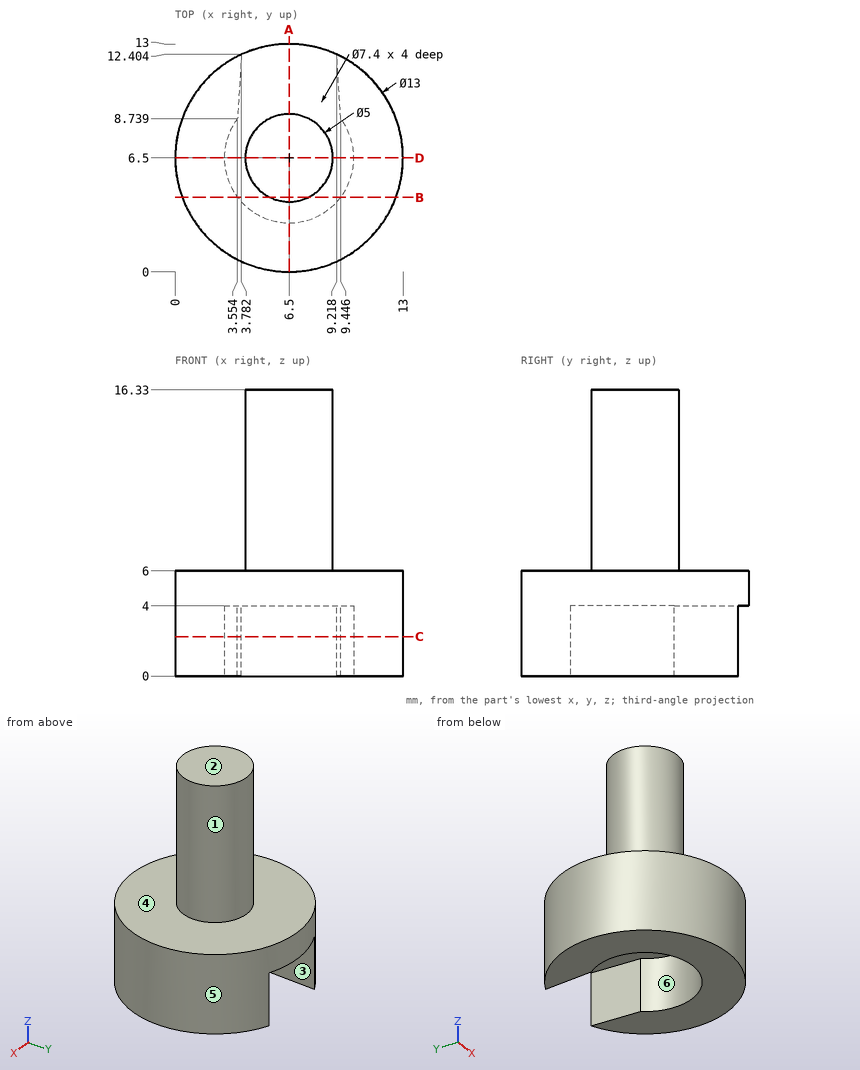
Answer from the drawing. Dimensions are ordinates in mm from the lowest x, y and z of the part. A direction names the side the tool comes from. Round coordinates to 2 decimals unless told otherwise and drop trailing zeros. Write each loop counter-clockwise with the first axis right and the second up, starting at its lowest first coordinate (ties: lowest second). Pieces come first, ordered by that corner, then holes. Notation, with made-up numbers: (85, 87.5) -> (115, 87.5) arc R18 ccw to (115, 94.5) -> close; hole circle Ø11 at (22, 68.25). An arc over 180 degrees is marked (long way). Write each question's results on one line, items separated by ' | '.
1) Flat-ended cylindrical pins translate along their axes: pin 1 (2 mm diameter, centred on x = 3, z = 5, fed in from +Y); pin 2 (1 mm diameter, centred on x = 3.5, y = 10.5, fed in from +Z); pin 3 (1.5 mm diameter, centred on x = 11, z = 13.5, fed in from +Y). Find the tip coordinate at first contact, or state that the pin passes through.
Findings:
pin 1: stops at y = 12.5 | pin 2: stops at z = 6 | pin 3: passes through
2) For a pull along X with two mould halves and no side action, classify the marked faces 1, 2 and 3 as +X half, -X half, draft (parallel to the pull), parting line (faces both ways), or undercut.
Findings:
face 1: parting line | face 2: draft | face 3: undercut
3) Which of the six approach directions +Z, -Z, +X, -X, +Y, -Y give full straight-line access (tool end or side, diameter ignored) to the marked faces 4, 5 and 6?
Findings:
face 4: +Z | face 5: +Z, -Z | face 6: -Z
4) Consider line 1 along X through (y, z) = (6.5, 1.75); line 2 along Z through (x, y) = (5.5, 0.75); line 3 along Y through (x, z) = (6.5, 1.5). Determine where each line is inside the solid, lowest interval first. Write a range as [from, to].
Findings:
line 1: x = [0, 2.8], [10.2, 13] | line 2: z = [0, 6] | line 3: y = [0, 2.8]
5) The part is cut by section C-C (z = 2.25). Write down the section's boundary in (x, y) (1 decimal).
Findings:
outline: (3.6, 8.7) -> (3.8, 12.4) arc R6.5 ccw (long way) to (9.2, 12.4) -> (9.4, 8.7) arc R3.7 cw (long way) to start
6) The part is cut by section D-D (y = 6.5). Write down the section's boundary in (x, z).
Findings:
outline: (0, 0) -> (2.8, 0) -> (2.8, 4) -> (10.2, 4) -> (10.2, 0) -> (13, 0) -> (13, 6) -> (9, 6) -> (9, 16.33) -> (4, 16.33) -> (4, 6) -> (0, 6) -> close
7) The part is cut by section A-A (x = 6.5). Write down the section's boundary in (y, z).
Findings:
outline: (0, 0) -> (2.8, 0) -> (2.8, 4) -> (13, 4) -> (13, 6) -> (9, 6) -> (9, 16.33) -> (4, 16.33) -> (4, 6) -> (0, 6) -> close
8) The part is cut by section B-B (y = 4.25). Write down the section's boundary in (x, z).
Findings:
outline: (0.4, 0) -> (3.56, 0) -> (3.56, 4) -> (9.44, 4) -> (9.44, 0) -> (12.6, 0) -> (12.6, 6) -> (7.59, 6) -> (7.59, 16.33) -> (5.41, 16.33) -> (5.41, 6) -> (0.4, 6) -> close
